Autodesk Inventor part; units mm, degrees
ref_plane "YZ Plane" through (0, 0, 0) normal (1, 0, 0) x (0, 1, 0)
ref_plane "XZ Plane" through (0, 0, 0) normal (0, 1, 0) x (-1, 0, 0)
ref_plane "XY Plane" through (0, 0, 0) normal (0, 0, 1) x (1, 0, 0)
sketch "Sketch1" plane through (0, 0, 0) normal (0, 0, 1) x (1, 0, 0)
  line L0 (-20.8392, 159.2122) -> (690.3608, 159.2122)
  line L1 (690.3608, 159.2122) -> (690.3608, -12.2378)
  line L2 (690.3608, -12.2378) -> (-20.8392, -12.2378)
  line L3 (-20.8392, -12.2378) -> (-20.8392, 159.2122)
  point P0 (0, 0)
  dimension "d0" = 171.45
  dimension "d1" = 711.2
extrude "Extrusion1" add sketch "Sketch1" along normal blind 19.05
sketch "Sketch2" plane through (0, 0, 19.05) normal (0, 0, 1) x (1, 0, 0)
  line L0 (690.3608, 159.2122) -> (690.3608, -12.2378)
  line L1 (-20.8392, -12.2378) -> (-20.8392, 159.2122)
  line L2 (690.3608, -12.2378) -> (-20.8392, -12.2378)
  line L3 (42.6608, 102.0622) -> (626.8608, 102.0622)
  line L4 (626.8608, 102.0622) -> (626.8608, -12.2378)
  line L5 (626.8608, -12.2378) -> (42.6608, -12.2378)
  line L6 (42.6608, -12.2378) -> (42.6608, 102.0622)
  line L7 (42.6608, 102.0622) -> (17.2608, -12.2378)
  line L8 (626.8608, 102.0622) -> (652.2608, -12.2378)
  point P0 (0, 0)
  dimension "d4" = 25.4
  dimension "d5" = 25.4
  dimension "d6" = 38.1
  dimension "d7" = 38.1
  dimension "d10" = 114.3
extrude "Extrusion2" cut sketch "Sketch2" against normal blind 19.05
properties part number "ridgidizer"
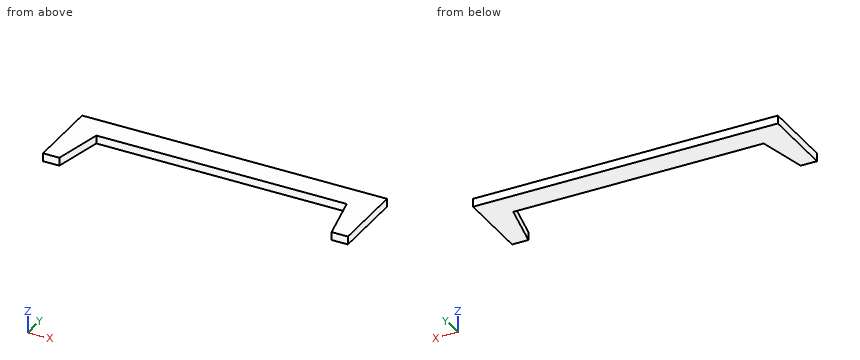
Geometry check sheet. Reference: the model listing, model coordinates, mm. Give positions to 0.01 mm unless a question says otherwise; leave off trailing zeros. Loops run counter-clockwise (first coordinate to the right, second up) from the corner with the lowest first, then second, coordinate; pieces in that order, holes last.
(1) Section check D-D on y = 22. Record the cut outline in (x, z), then the cut area to 3 significant figures.
From the geometry:
outline: (-20.84, 0) - (24.87, 0) - (24.87, 19.05) - (-20.84, 19.05) - close; (644.65, 0) - (690.36, 0) - (690.36, 19.05) - (644.65, 19.05) - close
area: 1,740 mm2
(2) Section check B-B on z = 7.25. Record the cut outline in (x, y).
From the geometry:
outline: (-20.84, -12.24) - (17.26, -12.24) - (42.66, 102.06) - (626.86, 102.06) - (652.26, -12.24) - (690.36, -12.24) - (690.36, 159.21) - (-20.84, 159.21) - close
(3) Depth check by flat-ended pin: pin 1 Ø2 at (x, z) = (369, 15) entering from -Y. Enter the tip coordinate at first touch or a pass-through.
From the geometry:
pin 1: stops at y = 102.06
(4) Section check C-C on x = 606.5. Record the cut outline in (y, z), then the cut area to 3 significant figures.
From the geometry:
outline: (102.06, 0) - (159.21, 0) - (159.21, 19.05) - (102.06, 19.05) - close
area: 1,090 mm2
(5) Section check A-A on y = 69. Record the cut outline in (x, z), then the cut area to 3 significant figures.
From the geometry:
outline: (-20.84, 0) - (35.31, 0) - (35.31, 19.05) - (-20.84, 19.05) - close; (634.21, 0) - (690.36, 0) - (690.36, 19.05) - (634.21, 19.05) - close
area: 2,140 mm2
(6) Thickness scan on L1, parallel to Y at x = 264, z = 7; L2, parallel to X at y = 86.5, z = 16.5; L3, parallel to X at y = 34, z = 18. Record the ranges inside material, lowest first.
From the geometry:
L1: y = 102.06 to 159.21
L2: x = -20.84 to 39.2, 630.32 to 690.36
L3: x = -20.84 to 27.54, 641.99 to 690.36
